Design review of the part built by this model. Coordinates are the model's own, in mm. Face numbers are marked on the shaded views. Give positions to 0.01 mm unless a question says otherwise; leave off trailing zeros. Loops run counter-clockwise (first coordinate to the right, second up) from the corner with the lowest first, then second, coordinate; pieces in that order, holes last. Notation, with made-up numbers: M -30,77 L -14,77 A17 ccw -14,88 Z; hole C 29.5,47.5 d7. An arc over 180 degrees is marked long. Answer as CSV lines item,"result".
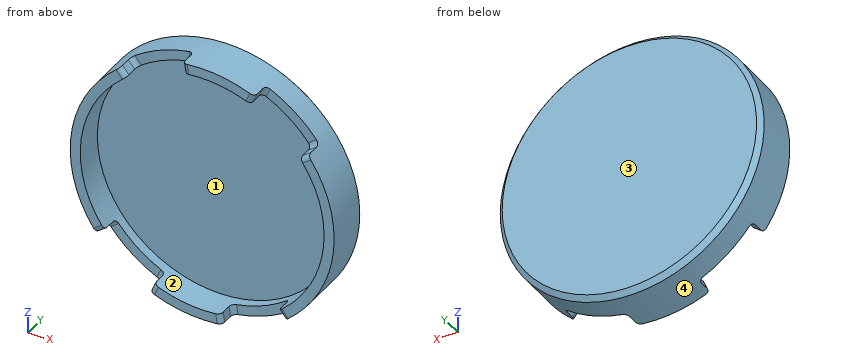
```python
from build123d import *

# Parameters (mm, degrees)
SKETCH1_R           = 13.75
BOSS_EXTRUDE1_DEPTH = 5
SKETCH2_R           = 12.7
CUT_EXTRUDE1_DEPTH  = 3
CHAMFER1_SIZE       = 0.5
CUT_EXTRUDE2_DEPTH  = 2
FILLET1_R           = 0.5


with BuildPart() as part:
    # Sketch1 → Boss-Extrude1 (new body)
    with BuildSketch(Plane(origin=(0, 0, 0), x_dir=(1, 0, 0), z_dir=(0, 1, 0))):
        Circle(SKETCH1_R)
    extrude(amount=BOSS_EXTRUDE1_DEPTH)

    # Sketch2 → Cut-Extrude1 (cut)
    with BuildSketch(Plane.XZ):
        Circle(SKETCH2_R)
    extrude(amount=-CUT_EXTRUDE1_DEPTH, mode=Mode.SUBTRACT)

    # Chamfer1
    chamfer1_edges = [part.edges().sort_by_distance(p)[0] for p in [
        (-13.75, 5, 0),
    ]]
    chamfer(chamfer1_edges, length=CHAMFER1_SIZE)

    # Sketch4 → Cut-Extrude2 (cut)
    with BuildSketch(Plane.XZ):
        with BuildLine():
            Line((8.580294574, -10.744349446), (7.92507208, -9.923871852))
            ThreePointArc((7.92507208, -9.923871852), (5.08654476, -11.636883707), (1.901377822, -12.556861167))
            Line((1.901377822, -12.556861167), (2.05857835, -13.595026855))
            ThreePointArc((2.05857835, -13.595026855), (5.507085863, -12.598988265), (8.580294574, -10.744349446))
        make_face()
        with BuildLine():
            Line((-5.442522653, -12.627012599), (-5.026911832, -11.662768001))
            ThreePointArc((-5.026911832, -11.662768001), (-7.874170442, -9.964308298), (-10.184817349, -7.586797451))
            Line((-10.184817349, -7.586797451), (-11.026869177, -8.214052358))
            ThreePointArc((-11.026869177, -8.214052358), (-8.525184534, -10.788129062), (-5.442522653, -12.627012599))
        make_face()
        with BuildLine():
            Line((-8.580294574, 10.744349446), (-7.92507208, 9.923871852))
            ThreePointArc((-7.92507208, 9.923871852), (-5.08654476, 11.636883707), (-1.901377822, 12.556861167))
            Line((-1.901377822, 12.556861167), (-2.05857835, 13.595026855))
            ThreePointArc((-2.05857835, 13.595026855), (-5.507085863, 12.598988265), (-8.580294574, 10.744349446))
        make_face()
        with BuildLine():
            Line((5.442522653, 12.627012599), (5.026911832, 11.662768001))
            ThreePointArc((5.026911832, 11.662768001), (7.874170442, 9.964308298), (10.184817349, 7.586797451))
            Line((10.184817349, 7.586797451), (11.026869177, 8.214052358))
            ThreePointArc((11.026869177, 8.214052358), (8.525184534, 10.788129062), (5.442522653, 12.627012599))
        make_face()
    extrude(amount=-CUT_EXTRUDE2_DEPTH, mode=Mode.SUBTRACT)

    # Fillet1
    fillet1_edges = [part.edges().sort_by_distance(p)[0] for p in [
        (5.234717242, 0, 12.1448903),
        (10.605843263, 2, 7.900424905),
        (5.234717242, 2, 12.1448903),
        (10.605843263, 0, 7.900424905),
        (-8.252683327, 0, 10.334110649),
        (-1.979978086, 2, 13.075944011),
        (-8.252683327, 2, 10.334110649),
        (-1.979978086, 0, 13.075944011),
        (-5.234717242, 0, -12.1448903),
        (-10.605843263, 2, -7.900424905),
        (-5.234717242, 2, -12.1448903),
        (-10.605843263, 0, -7.900424905),
        (8.252683327, 0, -10.334110649),
        (1.979978086, 2, -13.075944011),
        (8.252683327, 2, -10.334110649),
        (1.979978086, 0, -13.075944011),
    ]]
    fillet(fillet1_edges, radius=FILLET1_R)


solid = part.part
```
1. We need section C-C, the plane y = 3.35. Write out the cut boundary in (x, z).
Answer block:
outline,"C 0,0 d27.5"
2. We need section B-B, the plane z = 0. Write out the cut boundary in (x, y), plus the area to 4 significant figures.
Answer block:
outline,"M -13.75,0 L -12.7,0 L -12.7,3 L 12.7,3 L 12.7,0 L 13.75,0 L 13.75,4.5 L 13.25,5 L -13.25,5 L -13.75,4.5 Z"
area,"61.05 mm²"
3. The part is to be moulded in two halves that separate along X. For the marked faces 1, 2, 3 and 4, say which applies: pulls with the +X half, pulls with the -X half, needs draft (parallel to the pull), parting line crosses it, or undercut.
Answer block:
face 1,"undercut"
face 2,"undercut"
face 3,"needs draft"
face 4,"parting line crosses it"
4. To check wall thickness, follow L1, parallel to Z at x = 0, y = 1.15; L2, parallel to Y at x = -11, z = -1.75. State the ranges of each line that lie inside material, in increasing order. Write a range as [from, to].
Answer block:
L1,"[-13.75, -12.7], [12.7, 13.75]"
L2,"[3, 5]"
5. For P1, Ø1.5, axis at x = 8.5, y = 3.5, coming from the -Z side; P2, Ø1, axis at y = 3, z = 7, coming from the +X side; P3, Ø1.5, axis at y = 3, z = 10.5, coming from the +X side, all flat-tipped, find the tip position at first contact; note any pin that passes through.
Answer block:
P1,"z = -11.36"
P2,"x = 12.12"
P3,"x = 9.7"
6. We need section A-A, the plane x = 0. Write out the cut boundary in (y, z).
Answer block:
outline,"M 0,-13.75 L 4.5,-13.75 L 5,-13.25 L 5,13.25 L 4.5,13.75 L 0,13.75 L 0,12.7 L 3,12.7 L 3,-12.7 L 0,-12.7 Z"
